Build history of the part. All positions in model axes, mm. A direction names the side the tool comes from. Coordinates: 2 decimals unless noted, no trailing zeros. Write each loop counter-clockwise with the first axis right and the second up, starting at its lowest first coordinate (ties: lowest second). Pieces come first, ordered by that corner, then holes.
```python
from build123d import *

# Parameters (mm, degrees)
F0_W      = 69.343508
F0_H      = 47.200218
F1_DEPTH  = 5
F1_FACE_W = 69.343508
F1_FACE_H = 47.200218
F2_DEPTH  = 5
F3_W      = 69.343508
F3_H      = 8.242194
F5_DEPTH  = 7
F4_W      = 69.343508
F4_H      = 38.958024
F6_W      = 69.343508
F6_H      = 38.958024
F7_DEPTH  = 25


with BuildPart() as f1:
    # F0 (on Top) → F1 (new body)
    with BuildSketch(Plane.XY):
        Rectangle(F0_W, F0_H)
    extrude(amount=F1_DEPTH)

    # F1_face (on face) → F2 (join)
    with BuildSketch(Plane(origin=(0, 0, 0), x_dir=(1, 0, 0), z_dir=(0, 0, -1))):
        Rectangle(F1_FACE_W, F1_FACE_H)
    extrude(amount=F2_DEPTH)

    # F3 (on face) → F5 (join)
    with BuildSketch(Plane.XY.offset(5)):
        with Locations((0, -19.479012)):
            Rectangle(F3_W, F3_H)
    extrude(amount=F5_DEPTH)

    # F4 (on face) + F6 (on face) → F7 (join)
    with BuildSketch(Plane.XY.offset(5)):
        with Locations((0, 4.121097)):
            Rectangle(F4_W, F4_H)
    with BuildSketch(Plane.XY.offset(5)):
        with Locations((0, 4.121097)):
            Rectangle(F6_W, F6_H)
    extrude(amount=F7_DEPTH)


solid = f1.part
```
1. Flat gauge pins, fed straight in: pin 1 (2 mm diameter, centred on x = 16.5, z = 17, fed in from -Y); pin 2 (2.5 mm diameter, centred on x = 10, y = -20.5, fed in from +Z). Where does each tip first touch, or does it go through?
Computed values:
pin 1: stops at y = -15.36
pin 2: stops at z = 12
2. Saw through at B-B on y = -19.5. List the corners of the cut face in (x, z).
Computed values:
outline: (-34.67, -5) - (34.67, -5) - (34.67, 12) - (-34.67, 12) - close
3. Probe line 1 along Y through (x, z) = (5, 28). List the from-to ranges inside material, lowest first.
Computed values:
line 1: y = -15.36 to 23.6
4. Saw through at A-A on x = -8. List the corners of the cut face in (y, z), plus the area to 3 significant figures.
Computed values:
outline: (-23.6, -5) - (23.6, -5) - (23.6, 30) - (-15.36, 30) - (-15.36, 12) - (-23.6, 12) - close
area: 1,500 mm2
5. Saw through at C-C on z = 15.5. List the corners of the cut face in (x, y), plus the area to 3 significant figures.
Computed values:
outline: (-34.67, -15.36) - (34.67, -15.36) - (34.67, 23.6) - (-34.67, 23.6) - close
area: 2,700 mm2
6. 3-axis set-ups, long thin cutter, end or side, ignore diameter. For faces 1 (the face through (0, -23.6, 3)), 2 (the face through (0, -15.358, 21)): which of +Z, -Z, +X, -X, +Y, -Y reach the whole face in a straight line?
Computed values:
face 1: +Z, -Z, +X, -X, -Y
face 2: +Z, +X, -X, -Y
